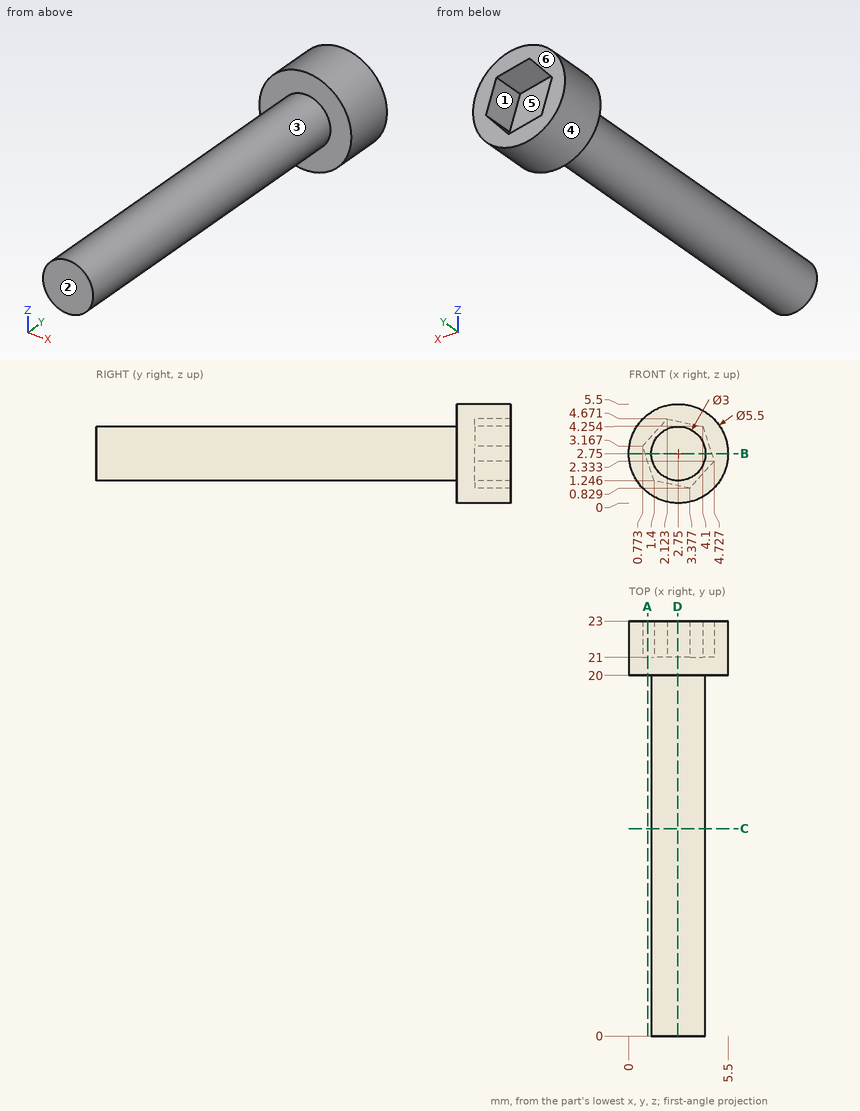
Geometry: see drawing. Coordinates: mm, zero at the bounding-box minimum. A direction names the side the tool comes from. Give positions to 0.01 mm unless a question says otherwise; leave off trailing zeros. Order: outer loops, then holes, each group sorted by start corner. A loop starts at its lowest first (then second) coordinate and runs counter-clockwise, first axis right, second up. Notation, with made-up numbers: (-31, 14.5) -> (-16, 14.5) arc R27 cw to (-16, 41.5) -> close; hole circle Ø3 at (46.5, 87.5). An arc over 180 degrees is marked (long way). Write each question's results on one line, items separated by ' | '. Start each with the question number.
1) Line query: line 1 (Y direction, x = 3.75, z = 1.55); line 2 (Y direction, x = 1.65, z = 2.25); line 3 (X direction, y = 22, z = 2.9) (1 decimal). Output: solid intervals per line, ascending. Write a range as from..to.
2) Draft query along Z for the marked faces 4, 5 and 6. Return one class per face: pulls with the +Z half, pulls with the -Z half, needs draft (parallel to the pull), parting line crosses it, or undercut.
3) Section C-C (y = 11.5). Return loops of the section in (x, z).
4) Set-up query: the marked faces 1, 2 and 3. Return all of +Z, -Z, +X, -X, +Y, -Y with unobstructed straight access to the full face (end or side cutting, diameter ignored); none if empty.
5) Section A-A (x = 1.05). Return loops of the section in (y, z).
6) First-contact query: pin 1 (1 mm diameter, centred on x = 3.5, y = 16.5, fed in from -Z); pin 2 (1.5 mm diameter, centred on x = 3, y = 11, fed in from +Z); pin 3 (1.5 mm diameter, centred on x = 1, y = 6, fed in from +Z). Flat tips, straight axial feed; report the tip coordinate or a pass-through.
7) Section D-D (x = 2.7). Return loops of the section in (y, z).
8) Section B-B (z = 2.75). Return loops of the section in (x, y).
Calculated:
1) line 1: 20..21 | line 2: 0..21 | line 3: 0..0.9, 4.5..5.5
2) face 4: parting line crosses it | face 5: undercut | face 6: needs draft
3) outline: circle Ø3 at (2.75, 2.75)
4) face 1: +Y | face 2: +Z, -Z, +X, -X, -Y | face 3: -Y
5) outline: (20, 0.59) -> (23, 0.59) -> (23, 2.32) -> (21, 2.32) -> (21, 3.48) -> (23, 3.48) -> (23, 4.91) -> (20, 4.91) -> close
6) pin 1: z = 1.27 | pin 2: z = 4.25 | pin 3: z = 3.87
7) outline: (0, 1.25) -> (20, 1.25) -> (20, 0) -> (23, 0) -> (23, 0.97) -> (21, 0.97) -> (21, 4.55) -> (23, 4.55) -> (23, 5.5) -> (20, 5.5) -> (20, 4.25) -> (0, 4.25) -> close
8) outline: (0, 20) -> (1.25, 20) -> (1.25, 0) -> (4.25, 0) -> (4.25, 20) -> (5.5, 20) -> (5.5, 23) -> (4.59, 23) -> (4.59, 21) -> (0.91, 21) -> (0.91, 23) -> (0, 23) -> close
